Design review of the part built by this model. Coordinates are the model's own, in mm. Give positions to 0.01 mm unless a question says otherwise; leave off trailing zeros. Loops run counter-clockwise (first coordinate to the right, second up) from the corner with the lowest first, then second, coordinate; pieces in that order, holes last. Notation, with made-up numbers: (78, 40) -> (121, 40) arc R21 cw to (121, 50) -> close; hole circle Ø7 at (47.5, 45.5). An arc over 180 degrees is marked (long way). Answer in a Markdown table with one row per item. Add a question column.
(1) For line 1 (X direction, y = -2, z = 6.5); line 2 (Z direction, x = 2.25, y = 1), list the stretches that pass through material, from the lowest coordinate up.
(2) For pin 1 (1.2 mm diameter, centred on y = -2, z = 5.5, fed in from +X); pin 2 (0.7 mm diameter, centred on y = 1.5, z = 8.5, fed in from -X); pin 3 (1.2 mm diameter, centred on x = -1.5, z = -7.5, fed in from -Y), all flat-tipped, find the tip position at first contact; note any pin that passes through.
(3) Consider section A-A on x = 0. Write out the cut boundary in (y, z).
(4) Consider section C-C on z = 11.5. Write out the cut boundary in (x, y), then the cut area to 3 significant figures.
Autodesk Inventor part; units mm, degrees
ref_plane "YZ Plane" through (0, 0, 0) normal (1, 0, 0) x (0, 1, 0)
ref_plane "XZ Plane" through (0, 0, 0) normal (0, 1, 0) x (-1, 0, 0)
ref_plane "XY Plane" through (0, 0, 0) normal (0, 0, 1) x (1, 0, 0)
sketch "Sketch1" plane through (0, 0, 0) normal (0, 0, 1) x (1, 0, 0)
  circle A0 centre (0, 0) radius 2.4 construction
  line L0 (-0.8, 2.2627) -> (-0.8, 0.8)
  line L1 (-0.8, 0.8) -> (-2.2627, 0.8)
  line L2 (-2.2627, -0.8) -> (-0.8, -0.8)
  line L3 (-0.8, -0.8) -> (-0.8, -2.2627)
  line L4 (0.8, -2.2627) -> (0.8, -0.8)
  line L5 (0.8, -0.8) -> (2.2627, -0.8)
  line L6 (2.2627, 0.8) -> (0.8, 0.8)
  line L7 (0.8, 0.8) -> (0.8, 2.2627)
  arc A1 (0.8, 2.2627) -> (-0.8, 2.2627) centre (0, 0) ccw
  arc A2 (-2.2627, 0.8) -> (-2.2627, -0.8) centre (0, 0) ccw
  arc A3 (-0.8, -2.2627) -> (0.8, -2.2627) centre (0, 0) ccw
  arc A4 (2.2627, -0.8) -> (2.2627, 0.8) centre (0, 0) ccw
  dimension "d0" = 4.8
  dimension "d1" = 1.6
extrude "Extrusion1" add sketch "Sketch1" along normal mid plane 40
sketch "Sketch2" plane through (0, 0, -20) normal (0, 0, -1) x (-1, 0, 0)
  line L0 (0.8, 0.8) -> (0.8, 2.2627)
  arc A0 (0.8, 2.2627) -> (-0.8, 2.2627) centre (0, 0) ccw
  line L1 (-0.8, 2.2627) -> (-0.8, 0.8)
  line L2 (-0.8, 0.8) -> (-2.2627, 0.8)
  arc A1 (-2.2627, 0.8) -> (-2.2627, -0.8) centre (0, 0) ccw
  line L3 (-2.2627, -0.8) -> (-0.8, -0.8)
  line L4 (-0.8, -0.8) -> (-0.8, -2.2627)
  arc A2 (-0.8, -2.2627) -> (0.8, -2.2627) centre (0, 0) ccw
  line L5 (0.8, -2.2627) -> (0.8, -0.8)
  line L6 (0.8, -0.8) -> (2.2627, -0.8)
  arc A3 (2.2627, -0.8) -> (2.2627, 0.8) centre (0, 0) ccw
  line L7 (2.2627, 0.8) -> (0.8, 0.8)
  circle A4 centre (0, 0) radius 3.2
  dimension "d7" = 6.4
extrude "Extrusion2" add sketch "Sketch2" against normal blind 0.8
fillet "Fillet1" radius 0.4 4 edges at (0, 2.4, 20) (-2.4, 0, 20) (0, -2.4, 20) (2.4, 0, 20)
fillet "Fillet1" radius 0.1 2 edges at (3.2, 0, -19.2) (3.2, 0, -20)
equation "\"d0\" = kd"
equation "\"d1\" = axlet"
equation "\"d2\" = 5 * lu"
equation "\"d7\" = tsd"
equation "\"d8\" = tsl"
equation "\"d4\" = tf"
equation "\"d10\" = lf"
properties part number "15462-ReddishBrown" material "ABS Plastic"
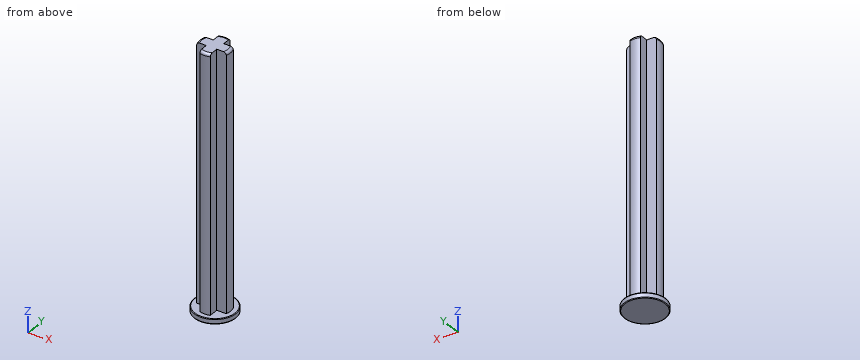
Values follow:
| question | item | result |
|---|---|---|
| 1 | line 1 | -0.8 to 0.8 |
| 1 | line 2 | -20 to -19.2 |
| 2 | pin 1 | x = 0.8 |
| 2 | pin 2 | x = -0.8 |
| 2 | pin 3 | y = -0.8 |
| 3 | outline | (-3.2, -19.9) arc R0.1 ccw to (-3.1, -20) -> (3.1, -20) arc R0.1 ccw to (3.2, -19.9) -> (3.2, -19.3) arc R0.1 ccw to (3.1, -19.2) -> (2.4, -19.2) -> (2.4, 19.6) arc R0.4 ccw to (2, 20) -> (-2, 20) arc R0.4 ccw to (-2.4, 19.6) -> (-2.4, -19.2) -> (-3.1, -19.2) arc R0.1 ccw to (-3.2, -19.3) -> close |
| 4 | outline | (-2.26, -0.8) -> (-0.8, -0.8) -> (-0.8, -2.26) arc R2.4 ccw to (0.8, -2.26) -> (0.8, -0.8) -> (2.26, -0.8) arc R2.4 ccw to (2.26, 0.8) -> (0.8, 0.8) -> (0.8, 2.26) arc R2.4 ccw to (-0.8, 2.26) -> (-0.8, 0.8) -> (-2.26, 0.8) arc R2.4 ccw to start |
| 4 | area | 12.5 mm2 |
